Autodesk Inventor part; units mm, degrees
ref_plane "StartOfTaper" through (-173.1851, -40.4973, 1.025) normal (0, 0, -1) x (-1, 0, 0)
ref_plane "EndOfTaper" through (-173.1851, -40.4973, 0) normal (0, 0, -1) x (-1, 0, 0)
ref_plane "ThisMuchIntoBezel" through (-173.1851, -40.4973, -2.4) normal (0, 0, -1) x (-1, 0, 0)
sketch "Sketch1" plane through (0, 0, 0) normal (0, 0, 1) x (1, 0, 0)
  circle A0 centre (-173.1851, -40.4973) radius 1.5
  point P0 (0, 0)
  dimension "d0" = 3
extrude "Extrusion1" add sketch "Sketch1" against normal blind 5
thread "Thread1"
sketch "Sketch2" plane through (-173.1851, -40.4973, 0) normal (0, 0, 1) x (1, 0, 0)
  circle A0 centre (0, 0) radius 2.525
  point P0 (173.1851, 40.4973)
  dimension "d5" = 5.05
extrude "Extrusion2" add sketch "Sketch2" along normal blind 1.82
chamfer "Chamfer1" distance 1.025 angle 45 1 edges at (-175.7101, -40.4973, 0)
sketch "Sketch3" plane through (-173.1851, -40.4973, 1.82) normal (0, 0, 1) x (1, 0, 0)
  line L0 (0, 1.5) -> (0, -1.5)
  line L1 (-1.5, 0) -> (1.5, 0)
  line L2 (-1.479, 0.25) -> (1.479, 0.25)
  line L3 (1.479, 0.25) -> (1.479, -0.25)
  line L4 (1.479, -0.25) -> (-1.479, -0.25)
  line L5 (-1.479, -0.25) -> (-1.479, 0.25)
  line L6 (-1.479, 0.25) -> (1.479, -0.25) construction
  line L7 (1.479, 0.25) -> (-1.479, -0.25) construction
  line L8 (0.25, 1.479) -> (-0.25, 1.479)
  line L9 (-0.25, 1.479) -> (-0.25, -1.479)
  line L10 (-0.25, -1.479) -> (0.25, -1.479)
  line L11 (0.25, -1.479) -> (0.25, 1.479)
  line L12 (0.25, 1.479) -> (-0.25, -1.479) construction
  line L13 (-0.25, 1.479) -> (0.25, -1.479) construction
  point P0 (173.1851, 40.4973)
  point P1 (0, 0)
  point P2 (-0.25, 0.25)
  point P3 (-0.25, -0.25)
  point P4 (0.25, -0.25)
  point P5 (0.25, 0.25)
  dimension "d12" = 0.5
  dimension "d13" = 0.5
extrude "Extrusion3" cut sketch "Sketch3" against normal blind 0.5
ref_plane "StartOfTaper" through (-173.1851, -40.4973, 1.025) normal (0, 0, -1) x (-1, 0, 0)
ref_plane "EndOfTaper" through (-173.1851, -40.4973, 0) normal (0, 0, -1) x (-1, 0, 0)
ref_plane "ThisMuchIntoBezel" through (-173.1851, -40.4973, -2.4) normal (0, 0, -1) x (-1, 0, 0)
properties part number "M3 Screw"
Check sheet for the modelled part. Datum: model origin and axes. Units: mm. A direction names the side the tool comes from. Coordinates: 2 decimals unless noted, no trailing zeros. Loops run counter-clockwise (first coordinate to the right, second up) from the corner with the lowest first, then second, coordinate; pieces in that order, holes last. Notation, with made-up numbers: (40, 18.5) -> (77, 18.5) arc R21 ccw to (77, 37.5) -> close; hole circle Ø9 at (26, 67.5). An arc over 180 degrees is marked (long way). Answer in a Markdown table with one row per item.
1. Access from +Z, -Z, +X, -X, +Y, -Y to the whole of each face (thin tool, end or side, straight path). Record for faces 1 (the face through (-171.8, -41.07, -2.46)), 2 (the face through (-172.7, -41, 1.82)).
Check values:
| item | result |
|---|---|
| face 1 | -Z |
| face 2 | +Z, +X, -X, +Y, -Y |
2. Sectioned sample at B-B, the plane z = -1.5. Record the boundary of the cut face in (x, y).
Check values:
| item | result |
|---|---|
| outline | circle Ø3 at (-173.19, -40.5) |
3. Go/stop test with flat-tipped pins: pin 1 (0.6 mm diameter, centred on y = -41, z = 1.5, fed in from -X); pin 2 (2 mm diameter, centred on y = -42, z = -4, fed in from +X); pin 3 (0.6 mm diameter, centred on x = -172, z = 1.5, fed in from +Y). Record where each tip stops, or that it passes through.
Check values:
| item | result |
|---|---|
| pin 1 | stops at x = -175.7 |
| pin 2 | stops at x = -171.77 |
| pin 3 | stops at y = -38.13 |
4. Sectioned sample at A-A, the plane z = 0.25. Record the boundary of the cut face in (x, y), then the cut area to 3 significant figures.
Check values:
| item | result |
|---|---|
| outline | circle Ø3.5 at (-173.19, -40.5) |
| area | 9.63 mm2 |
5. Material ranges on line 1 along Z through (x, y) = (-173.3, -41.8); line 2 along X through (y, z) = (-40.3, 1.75); line 3 along Z through (x, y) = (-173.55, -42.7), recorded low to high. Write a range as [from, to].
Check values:
| item | result |
|---|---|
| line 1 | z = [-5, 1.32] |
| line 2 | x = [-175.7, -174.66], [-171.71, -170.67] |
| line 3 | z = [0.73, 1.82] |
6. Release check for a two-part mould opening along X. For faces 3 (the face through (-173.3, -40.5, 1.32)), 4 (the face through (-173, -40, -5)), 5 (the face through (-175.05, -42.2, 1.42)) record: released by +X, released by -X, zero draft, split by the parting line, or undercut.
Check values:
| item | result |
|---|---|
| face 3 | undercut |
| face 4 | zero draft |
| face 5 | split by the parting line |
